Could you check a few things on this model? Use its own coordinates, in mm. A direction names the side the tool comes from. Give positions to 0.01 mm unless a question says otherwise; leave off trailing zeros. Write each loop counter-clockwise with the first axis right and the second up, starting at its lowest first coordinate (ties: lowest second). Pieces come first, ordered by that corner, then holes. Notation, with made-up numbers: M 0,-32 L 7,-32 A18 cw 7,1 Z; hole C 5,23.5 d6. An arc over 180 degrees is marked long. Use one line per item in the form item = value.
Autodesk Inventor part; units mm, degrees
ref_plane "YZ Plane" through (0, 0, 0) normal (1, 0, 0) x (0, 1, 0)
ref_plane "XZ Plane" through (0, 0, 0) normal (0, 1, 0) x (-1, 0, 0)
ref_plane "XY Plane" through (0, 0, 0) normal (0, 0, 1) x (1, 0, 0)
sketch "Sketch1" plane through (0, 0, 0) normal (0, 1, 0) x (-1, 0, 0)
  circle A0 centre (0, 0) radius 4
  circle A1 centre (0, 0) radius 8
  dimension "d0" = 8
  dimension "d1" = 16
extrude "Extrusion1" add sketch "Sketch1" along normal blind 5
sketch "Sketch2" plane through (0, 5, 0) normal (0, 1, 0) x (1, 0, 0)
  circle A0 centre (0, 0) radius 8
  circle A1 centre (0, 0) radius 4
  circle A2 centre (0, 0) radius 5
  circle A3 centre (0, 0) radius 6.5
  dimension "d4" = 10
  dimension "d5" = 13
extrude "Extrusion2" cut sketch "Sketch2" against normal blind 0.2 contours A3
sketch "Sketch3" plane through (0, 0, 0) normal (0, -1, 0) x (1, 0, 0)
  circle A0 centre (0, 0) radius 5
  circle A1 centre (0, 0) radius 6.5
extrude "Extrusion3" cut sketch "Sketch3" against normal blind 0.2
properties part number "bearing_8_16_5"
1) Thinking about a two-plate mould opening in Z: for faces 1 (the cylindrical face through (1.73, 2.46, 7.81)), 2 (the cylindrical face through (0.867, 2.465, 3.905)), 3 (the flat face through (0, 5, 7)), which applies, released by +Z, released by -Z, zero draft, split by the parting line, or undercut?
Checked values:
face_1 = split by the parting line
face_2 = undercut
face_3 = zero draft
2) For pin 1 Ø5 at (x, z) = (-3, -2.5) entering from -Y; pin 2 Ø1.5 at (x, z) = (-1, 1) entering from +Y; pin 3 Ø3 at (x, y) = (-4, 3.5) entering from -Z; pin 4 Ø3 at (y, z) = (3.5, -6.5) entering from -X (3 decimals), each with a flat end and sliding along its axis, tell me the tip position at first contact or that it passes through.
Checked values:
pin_1 = 0
pin_2 = through
pin_3 = -7.6
pin_4 = -6.245
3) I want a section at C-C, the plane y = 4.6. Please give me the cut outline in (x, z).
Checked values:
outline = C 0,0 d16; hole C 0,0 d8
4) I want a section at D-D, the plane z = 4.25. Please give me the cut outline in (x, y).
Checked values:
outline = M -6.78,0 L -4.92,0 L -4.92,0.2 L -2.63,0.2 L -2.63,0 L 2.63,0 L 2.63,0.2 L 4.92,0.2 L 4.92,0 L 6.78,0 L 6.78,5 L 4.92,5 L 4.92,4.8 L 2.63,4.8 L 2.63,5 L -2.63,5 L -2.63,4.8 L -4.92,4.8 L -4.92,5 L -6.78,5 Z
5) I want a section at B-B, the plane x = 0. Please give me the cut outline in (y, z), plus the area to 3 significant figures.
Checked values:
outline = M 0,-8 L 5,-8 L 5,-6.5 L 4.8,-6.5 L 4.8,-5 L 5,-5 L 5,-4 L 0,-4 L 0,-5 L 0.2,-5 L 0.2,-6.5 L 0,-6.5 Z; M 0,4 L 5,4 L 5,5 L 4.8,5 L 4.8,6.5 L 5,6.5 L 5,8 L 0,8 L 0,6.5 L 0.2,6.5 L 0.2,5 L 0,5 Z
area = 38.8 mm2
6) If I drill on L1, parallel to Z at x = 0, y = 0.15; L2, parallel to Z at x = 0, y = 3.15; L3, parallel to Y at x = 3.5, z = -4.25, over which ranges is the centre line in solid material (lowest first)?
Checked values:
L1 = -8 to -6.5, -5 to -4, 4 to 5, 6.5 to 8
L2 = -8 to -4, 4 to 8
L3 = 0.2 to 4.8
7) For faces 4 (the flat face through (2, 0.2, -5)), 5 (the flat face through (0, 0, 7)), 6 (the flat face through (2, 4.8, 5)), which set-ups out of +Z, -Z, +X, -X, +Y, -Y let a thin tool reach every point of the face, with its end or its side?
Checked values:
face_4 = -Y
face_5 = +Z, -Z, +X, -X, -Y
face_6 = +Y
8) I want a section at A-A, the plane z = 0. Please give me the cut outline in (x, y), plus the area to 3 significant figures.
Checked values:
outline = M -8,0 L -6.5,0 L -6.5,0.2 L -5,0.2 L -5,0 L -4,0 L -4,5 L -5,5 L -5,4.8 L -6.5,4.8 L -6.5,5 L -8,5 Z; M 4,0 L 5,0 L 5,0.2 L 6.5,0.2 L 6.5,0 L 8,0 L 8,5 L 6.5,5 L 6.5,4.8 L 5,4.8 L 5,5 L 4,5 Z
area = 38.8 mm2
